Geometry check sheet. Reference: the model listing, model coordinates, mm. A direction names the side the tool comes from. Coordinates: 2 decimals unless noted, no trailing zeros. Order: outer loops, then holes, each group sorted by start corner. A loop starts at its lowest first (then second) coordinate and runs counter-clockwise, first axis right, second up. Notation, with made-up numbers: (47, -14) - (53, -14) arc R22 cw to (53, 25) - close; hole circle Ø4 at (40, 83.25). An arc over 180 degrees is marked (long way). Put each result on its own line as item: value.
from build123d import *

# Parameters (mm, degrees)
F1_DEPTH     = 7.5
F2_DEPTH     = 7.5
F3_DEPTH     = 4.5
F4_SIZE      = 2
F5_T1_DEPTH  = 6.7433659759
F5_T4_ANGLE  = 220.4864882976
F5_T6_ANGLE  = 220.4864882976
F5_T10_ANGLE = 220.4864882976
F5_T15_ANGLE = 220.4864882976
F5_T20_ANGLE = 220.4864882976
F5_T25_ANGLE = 220.4864882976


# Not quite as in the source:
# - a fillet or chamfer that OpenCascade refuses, or shapes differently, is made with other operations: its cross-section is extruded or revolved along the edge and cut away or added


with BuildPart() as f1:
    # F0 (on Top) → F1 (new body)
    with BuildSketch(Plane.XY):
        with BuildLine():
            ThreePointArc((0.8, -3.6636730203), (2.9208303614, -2.3518609653), (3.75, 0))
            ThreePointArc((3.75, 0), (2.9208303614, 2.3518609653), (0.8, 3.6636730203))
            Line((0.8, 3.6636730203), (0.8, -3.6636730203))
        make_face()
        with BuildLine():
            Line((0.8, -3.6636730203), (0.8, 3.6636730203))
            ThreePointArc((0.8, 3.6636730203), (0, 3.75), (-0.8, 3.6636730203))
            Line((-0.8, 3.6636730203), (-0.8, -3.6636730203))
            ThreePointArc((-0.8, -3.6636730203), (0, -3.75), (0.8, -3.6636730203))
        make_face()
        with BuildLine():
            Line((-0.8, -3.6636730203), (-0.8, 3.6636730203))
            ThreePointArc((-0.8, 3.6636730203), (-3.75, 0), (-0.8, -3.6636730203))
        make_face()
    extrude(amount=-F1_DEPTH)

    # F0 (on Top) → F2 (join)
    with BuildSketch(Plane.XY):
        with BuildLine():
            ThreePointArc((0.8, -3.6636730203), (2.9208303614, -2.3518609653), (3.75, 0))
            ThreePointArc((3.75, 0), (2.9208303614, 2.3518609653), (0.8, 3.6636730203))
            Line((0.8, 3.6636730203), (0.8, -3.6636730203))
        make_face()
        with BuildLine():
            Line((0.8, -3.6636730203), (0.8, 3.6636730203))
            ThreePointArc((0.8, 3.6636730203), (0, 3.75), (-0.8, 3.6636730203))
            Line((-0.8, 3.6636730203), (-0.8, -3.6636730203))
            ThreePointArc((-0.8, -3.6636730203), (0, -3.75), (0.8, -3.6636730203))
        make_face()
        with BuildLine():
            Line((-0.8, -3.6636730203), (-0.8, 3.6636730203))
            ThreePointArc((-0.8, 3.6636730203), (-3.75, 0), (-0.8, -3.6636730203))
        make_face()
        with BuildLine():
            ThreePointArc((-0.8, 3.6636730203), (0, 3.75), (0.8, 3.6636730203))
            Line((0.8, 3.6636730203), (0.8, 4.95))
            Line((0.8, 4.95), (-0.8, 4.95))
            Line((-0.8, 4.95), (-0.8, 3.6636730203))
        make_face()
        with BuildLine():
            Line((0.8, -4.95), (0.8, -3.6636730203))
            ThreePointArc((0.8, -3.6636730203), (0, -3.75), (-0.8, -3.6636730203))
            Line((-0.8, -3.6636730203), (-0.8, -4.95))
            Line((-0.8, -4.95), (0.8, -4.95))
        make_face()
    extrude(amount=F2_DEPTH)

    # F0 (on Top) → F3 (join)
    with BuildSketch(Plane.XY):
        with BuildLine():
            ThreePointArc((0.8, 3.6636730203), (2.9208303614, 2.3518609653), (3.75, 0))
            ThreePointArc((3.75, 0), (2.9208303614, -2.3518609653), (0.8, -3.6636730203))
            Line((0.8, -3.6636730203), (0.8, -4.95))
            ThreePointArc((0.8, -4.95), (3.8179761524, -3.2504704428), (5.0142297514, 0))
            ThreePointArc((5.0142297514, 0), (3.8179761524, 3.2504704428), (0.8, 4.95))
            Line((0.8, 4.95), (0.8, 3.6636730203))
        make_face()
        with BuildLine():
            Line((0.8, -4.95), (0.8, -3.6636730203))
            ThreePointArc((0.8, -3.6636730203), (0, -3.75), (-0.8, -3.6636730203))
            Line((-0.8, -3.6636730203), (-0.8, -4.95))
            Line((-0.8, -4.95), (0.8, -4.95))
        make_face()
        with BuildLine():
            ThreePointArc((-0.8, -3.6636730203), (-3.75, 0), (-0.8, 3.6636730203))
            Line((-0.8, 3.6636730203), (-0.8, 4.95))
            ThreePointArc((-0.8, 4.95), (-5.0142297514, 0), (-0.8, -4.95))
            Line((-0.8, -4.95), (-0.8, -3.6636730203))
        make_face()
        with BuildLine():
            ThreePointArc((-0.8, 3.6636730203), (0, 3.75), (0.8, 3.6636730203))
            Line((0.8, 3.6636730203), (0.8, 4.95))
            Line((0.8, 4.95), (-0.8, 4.95))
            Line((-0.8, 4.95), (-0.8, 3.6636730203))
        make_face()
    extrude(amount=-F3_DEPTH)

    # F4
    f4_edges = [f1.edges().sort_by_distance(p)[0] for p in [
        (0.8, -3.663673, -7.5),
    ]]
    chamfer(f4_edges, length=F4_SIZE)

    # F5: chamfer of 1 on 6 edges, made by hand

    # F5_s2 → F5_t1 (cut)
    with BuildSketch(Plane.YZ.offset(-3.371682988)):
        Polygon((-3.95, -4.5), (-4.95, -3.5), (-4.95, -4.5), align=None)
        Polygon((3.95, -4.5), (4.95, -3.5), (4.95, -4.5), align=None)
    extrude(amount=F5_T1_DEPTH, mode=Mode.SUBTRACT)

    # F5_s3 → F5_t4 (revolve, cut)
    with BuildSketch(Plane(origin=(0, 0, 0), x_dir=(0, 0, 1), z_dir=(0.9382321407, -0.3460064308, 0))):
        Polygon((-4.5, -4.0142297514), (-3.5, -5.0142297514), (-4.5, -5.0142297514), align=None)
    revolve(axis=Axis((0, 0, -4.5), (0, 0, 1)), revolution_arc=F5_T4_ANGLE, mode=Mode.SUBTRACT)

    # F5_s5 → F5_t6 (revolve, cut)
    with BuildSketch(Plane(origin=(0, 0, 0), x_dir=(0, 0, 1), z_dir=(-0.9382321407, 0.3460064308, 0))):
        Polygon((-4.5, -4.0142297514), (-3.5, -5.0142297514), (-4.5, -5.0142297514), align=None)
    revolve(axis=Axis((0, 0, -4.5), (0, 0, 1)), revolution_arc=F5_T6_ANGLE, mode=Mode.SUBTRACT)


with BuildPart() as f5_tool8:
    # F5_s9 → F5_t10 (revolve)
    with BuildSketch(Plane(origin=(0, 0, 0), x_dir=(0, 0, 1), z_dir=(0.9382321407, -0.3460064308, 0))):
        Polygon((-1, -5.0142297514), (0, -4.0142297514), (0, -5.0142297514), align=None)
    revolve(axis=Axis((0, 0, 0), (0, 0, 1)), revolution_arc=F5_T10_ANGLE)

    split(bisect_by=Plane.YZ.offset(0.8), keep=Keep.TOP)


with BuildPart() as f1_1:
    add(f1.part)

    # F5_t7: cut F5_tool8
    add(f5_tool8.part, mode=Mode.SUBTRACT)


with BuildPart() as f5_tool13:
    # F5_s14 → F5_t15 (revolve)
    with BuildSketch(Plane(origin=(0, 0, 0), x_dir=(0, 0, 1), z_dir=(0.9382321407, -0.3460064308, 0))):
        Polygon((-1, -5.0142297514), (0, -4.0142297514), (0, -5.0142297514), align=None)
    revolve(axis=Axis((0, 0, 0), (0, 0, 1)), revolution_arc=F5_T15_ANGLE)

    split(bisect_by=Plane.YZ.offset(-0.8), keep=Keep.BOTTOM)


with BuildPart() as f1_2:
    add(f1_1.part)

    # F5_t12: cut F5_tool13
    add(f5_tool13.part, mode=Mode.SUBTRACT)


with BuildPart() as f5_tool18:
    # F5_s19 → F5_t20 (revolve)
    with BuildSketch(Plane(origin=(0, 0, 0), x_dir=(0, 0, 1), z_dir=(-0.9382321407, 0.3460064308, 0))):
        Polygon((-1, -5.0142297514), (0, -4.0142297514), (0, -5.0142297514), align=None)
    revolve(axis=Axis((0, 0, 0), (0, 0, 1)), revolution_arc=F5_T20_ANGLE)

    split(bisect_by=Plane.YZ.offset(-0.8), keep=Keep.BOTTOM)


with BuildPart() as f1_3:
    add(f1_2.part)

    # F5_t17: cut F5_tool18
    add(f5_tool18.part, mode=Mode.SUBTRACT)


with BuildPart() as f5_tool23:
    # F5_s24 → F5_t25 (revolve)
    with BuildSketch(Plane(origin=(0, 0, 0), x_dir=(0, 0, 1), z_dir=(-0.9382321407, 0.3460064308, 0))):
        Polygon((-1, -5.0142297514), (0, -4.0142297514), (0, -5.0142297514), align=None)
    revolve(axis=Axis((0, 0, 0), (0, 0, 1)), revolution_arc=F5_T25_ANGLE)

    split(bisect_by=Plane.YZ.offset(0.8), keep=Keep.TOP)


with BuildPart() as f1_4:
    add(f1_3.part)

    # F5_t22: cut F5_tool23
    add(f5_tool23.part, mode=Mode.SUBTRACT)


solid = f1_4.part
Q1. Draft check along Y on faces 1 (the flat face through (0, -4.95, 2)), 2 (the flat face through (-0.8, -4, 3)), 3 (the cylindrical face through (-3.75, 0.07, 3.7)). Enter one of: pulls with the +Y half, pulls with the -Y half, needs draft (parallel to the pull), parting line crosses it, or undercut.
Answer block:
face 1: pulls with the -Y half
face 2: needs draft
face 3: parting line crosses it
Q2. Section check A-A on z = 0.75. Record the boundary of the cut face in (x, y).
Answer block:
outline: (-0.8, -4.95) - (0.8, -4.95) - (0.8, -3.66) arc R3.75 ccw to (0.8, 3.66) - (0.8, 4.95) - (-0.8, 4.95) - (-0.8, 3.66) arc R3.75 ccw to (-0.8, -3.66) - close
Q3. Section check C-C on z = -2.75. Record the boundary of the cut face in (x, y), then the cut area to 3 significant figures.
Answer block:
outline: (-0.8, -4.95) - (0.8, -4.95) arc R5.01 ccw to (0.8, 4.95) - (-0.8, 4.95) arc R5.01 ccw to start
area: 78.9 mm^2
Q4. Thickness scan on L1, parallel to X at y = -4.25, z = 2.5; L2, parallel to X at y = -1, z = -1.25; L3, parallel to Y at x = 1.75, z = -0.25. Record the ranges inside material, lowest first. Write a range as [from, to].
Answer block:
L1: x = [-0.8, 0.8]
L2: x = [-4.91, 4.91]
L3: y = [-3.89, 3.89]
Q5. Depth check by flat-ended pin: pin 1 Ø3 at (x, z) = (-4, -4.5) entering from -Y; pin 2 Ø1.4 at (y, z) = (4, 3) entering from +X; pin 3 Ø1 at (x, z) = (-3, -1) entering from +Y. Enter the tip coordinate at first touch or a pass-through.
Answer block:
pin 1: stops at y = -4.1
pin 2: stops at x = 1.78
pin 3: stops at y = 4.35
Q6. Section check B-B on x = 0. Record the boundary of the cut face in (y, z).
Answer block:
outline: (-4.95, -3.5) - (-3.95, -4.5) - (-3.75, -4.5) - (-3.75, -5.5) - (-1.75, -7.5) - (1.75, -7.5) - (3.75, -5.5) - (3.75, -4.5) - (3.95, -4.5) - (4.95, -3.5) - (4.95, 7.5) - (-4.95, 7.5) - close
Q7. Access from +Z, -Z, +X, -X, +Y, -Y to the whole of each face (thin tool, end or side, straight path). Record for faces 4 (the cylindrical face through (-5.013, 0.099, -2.232)), 5 (the flat face through (-0.8, 4, 3)), 6 (the flat face through (0.8, -4, 3)).
Answer block:
face 4: +Z, -Z, -X
face 5: +Z, -X, +Y
face 6: +Z, +X, -Y
